Geometry check sheet. Reference: the model listing, model coordinates, mm. A direction names the side the tool comes from. Coordinates: 2 decimals unless noted, no trailing zeros. Order: outer loops, then holes, each group sorted by start corner. A loop starts at its lowest first (then second) coordinate and runs counter-clockwise, first axis right, second up. Notation, with made-up numbers: (75.5, 57.25) -> (116.5, 57.25) arc R13 cw to (116.5, 73.25) -> close; hole circle Ø4 at (67, -6). An arc over 180 degrees is marked (long way). Answer in a Markdown table with one row per item. Add a question column.
```python
from build123d import *

# Parameters (mm, degrees)
F0_W     = 914.4
F0_H     = 914.4
F1_DEPTH = 25.4
F2_R     = 12.7
F3_DEPTH = 38.1
F5_D     = 12.7


with BuildPart() as f1:
    # F0 (on Right) → F1 (new body)
    with BuildSketch(Plane.YZ):
        Rectangle(F0_W, F0_H)
    extrude(amount=F1_DEPTH)

    # F2 (on face) → F3 (join)
    with BuildSketch(Plane.YZ.offset(25.4)):
        Circle(F2_R)
    extrude(amount=F3_DEPTH)

    # F5 (through all)
    with Locations(Plane.YZ.offset(25.4)):
        with Locations((155.575, 112.7125), (219.075, 112.7125), (155.575, -112.7125), (219.075, -112.7125)):
            Hole(F5_D / 2)


solid = f1.part
```
(1) Cross-section at D-D (y = 246.5). Enter the section's corners in (x, z).
(2) Go/stop test with flat-tipped pins: P1, Ø10, axis at y = -287, z = -158, coming from the +X side; P2, Ø7.5, axis at y = 155.57, z = 112.71, coming from the +X side; P3, Ø6, axis at x = 46.5, z = -8.5, coming from the -Y side. Record where each tip stops, or that it passes through.
(3) Cross-section at A-A (z = 0). Enter the section's corners in (x, y).
(4) Cross-section at C-C (x = 47). Enter the section's corners in (y, z).
(5) Access from +Z, -Z, +X, -X, +Y, -Y to the whole of each face (thin tool, end or side, straight path). Record for faces 1 (the face through (13, -6, 457.2)), 2 (the face through (44.18, -2.75, -12.4)).
(6) Scan line: line 1 along X through (y, z) = (335.5, -230.5). Record every from-to range of solid material in increasing order.
Checks:
| question | item | result |
|---|---|---|
| 1 | outline | (0, -457.2) -> (25.4, -457.2) -> (25.4, 457.2) -> (0, 457.2) -> close |
| 2 | P1 | x = 25.4 |
| 2 | P2 | through |
| 2 | P3 | y = -11.45 |
| 3 | outline | (0, -457.2) -> (25.4, -457.2) -> (25.4, -12.7) -> (63.5, -12.7) -> (63.5, 12.7) -> (25.4, 12.7) -> (25.4, 457.2) -> (0, 457.2) -> close |
| 4 | outline | circle Ø25.4 at (0, 0) |
| 5 | face 1 | +Z, +X, -X, +Y, -Y |
| 5 | face 2 | +X |
| 6 | line 1 | 0 to 25.4 |
